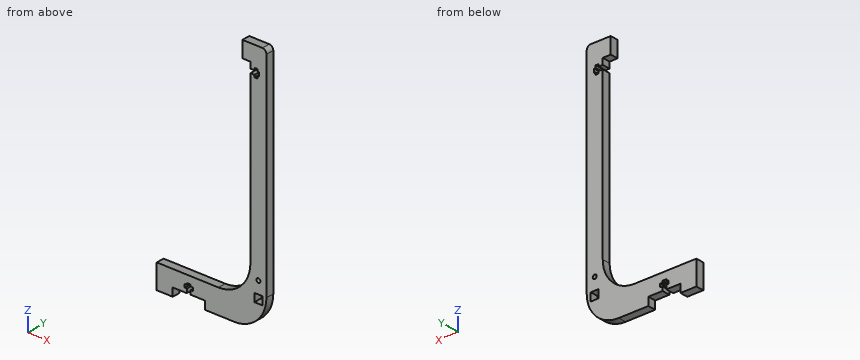
from build123d import *

# Parameters (mm, degrees)
SKETCH1_R           = 1.5875
BOSS_EXTRUDE1_DEPTH = 6.35


with BuildPart() as part:
    # Sketch1 → Boss-Extrude1 (new body)
    with BuildSketch(Plane(origin=(0, 0, 0), x_dir=(1, 0, 0), z_dir=(0, 1, 0))):
        with BuildLine():
            Line((7.882687692, 29.208698466), (-41.012312308, 29.208698466))
            Line((-41.012312308, 29.208698466), (-41.012312308, 48.258698466))
            Line((-41.012312308, 48.258698466), (-28.312312308, 48.258698466))
            Line((-28.312312308, 48.258698466), (-28.312312308, 41.908698466))
            Line((-28.312312308, 41.908698466), (-17.136241986, 41.908698466))
            Line((-17.136241986, 41.908698466), (-17.136241986, 38.733698466))
            Line((-17.136241986, 38.733698466), (-18.888841986, 38.733698466))
            Line((-18.888841986, 38.733698466), (-18.888841986, 36.193698466))
            Line((-18.888841986, 36.193698466), (-17.136241986, 36.193698466))
            Line((-17.136241986, 36.193698466), (-17.136241986, 34.923698466))
            Line((-17.136241986, 34.923698466), (-14.08838263, 34.923698466))
            Line((-14.08838263, 34.923698466), (-14.08838263, 36.193698466))
            Line((-14.08838263, 36.193698466), (-12.33578263, 36.193698466))
            Line((-12.33578263, 36.193698466), (-12.33578263, 38.733698466))
            Line((-12.33578263, 38.733698466), (-14.08838263, 38.733698466))
            Line((-14.08838263, 38.733698466), (-14.08838263, 41.908698466))
            Line((-14.08838263, 41.908698466), (-2.912312308, 41.908698466))
            Line((-2.912312308, 41.908698466), (-2.912312308, 48.258698466))
            Line((-2.912312308, 48.258698466), (20.582687692, 48.258698466))
            ThreePointArc((20.582687692, 48.258698466), (38.543199934, 40.819210709), (45.982687692, 22.858698466))
            Line((45.982687692, 22.858698466), (45.982687692, -143.587501534))
            ThreePointArc((45.982687692, -143.587501534), (45.052751722, -145.832565564), (42.807687692, -146.762501534))
            Line((42.807687692, -146.762501534), (33.282687692, -146.762501534))
            Line((33.282687692, -146.762501534), (26.932687692, -146.762501534))
            Line((26.932687692, -146.762501534), (26.932687692, -134.062501534))
            Line((26.932687692, -134.062501534), (33.282687692, -134.062501534))
            Line((33.282687692, -134.062501534), (33.282687692, -129.236431212))
            Line((33.282687692, -129.236431212), (36.457687692, -129.236431212))
            Line((36.457687692, -129.236431212), (36.457687692, -130.989031212))
            Line((36.457687692, -130.989031212), (38.997687692, -130.989031212))
            Line((38.997687692, -130.989031212), (38.997687692, -129.236431212))
            Line((38.997687692, -129.236431212), (40.267687692, -129.236431212))
            Line((40.267687692, -129.236431212), (40.267687692, -126.188571855))
            Line((40.267687692, -126.188571855), (38.997687692, -126.188571855))
            Line((38.997687692, -126.188571855), (38.997687692, -124.435971855))
            Line((38.997687692, -124.435971855), (36.457687692, -124.435971855))
            Line((36.457687692, -124.435971855), (36.457687692, -126.188571855))
            Line((36.457687692, -126.188571855), (33.282687692, -126.188571855))
            Line((33.282687692, -126.188571855), (33.282687692, -121.362501534))
            Line((33.282687692, -121.362501534), (33.282687692, 3.808698466))
            ThreePointArc((33.282687692, 3.808698466), (25.843199934, 21.769210709), (7.882687692, 29.208698466))
        make_face()
        with Locations(Location((39.632687692, 13.333698466, 0), (0, 0, 270))):
            Circle(SKETCH1_R, mode=Mode.SUBTRACT)
        Polygon((39.632687692, 29.208698466), (42.807687692, 29.208698466), (42.807687692, 22.858698466), (36.457687692, 22.858698466), (36.457687692, 29.208698466), align=None, mode=Mode.SUBTRACT)
    extrude(amount=BOSS_EXTRUDE1_DEPTH)


solid = part.part
Verification items for the finished model (mm, model axes). Coordinates: 2 decimals unless noted, no trailing zeros. Loops run counter-clockwise (first coordinate to the right, second up) from the corner with the lowest first, then second, coordinate; pieces in that order, holes last. Notation, with made-up numbers: (55.5, 85) -> (98.5, 85) arc R22 ccw to (98.5, 95) -> close; hole circle Ø9 at (-24, -22). An arc over 180 degrees is marked (long way). Answer as CSV lines item,"result".
1) Thickness scan on L1, parallel to Z at x = 40, y = 2; L2, parallel to Z at x = -14, y = 4.75; L3, parallel to Z at x = 28.5, y = 4.75. Record the ranges inside material, lowest first. Write a range as from..to.
Found:
L1,"z = -39.23..-29.21, -22.86..-14.88, -11.79..126.19, 129.24..146.76"
L2,"z = -41.91..-38.73, -36.19..-29.21"
L3,"z = -46.99..-18.64, 134.06..146.76"
2) Depth check by flat-ended pin: pin 1 (1 mm diameter, centred on y = 5, z = 62.5, fed in from -X); pin 2 (1.5 mm diameter, centred on x = -16, y = 2, fed in from -Z); pin 3 (0.9 mm diameter, centred on x = -13, y = 4, fed in from +Z); pin 4 (6 mm diameter, centred on x = -22, z = -26, fed in from +Y). Enter the tip coordinate at first touch or a pass-through.
Found:
pin 1,"stops at x = 33.28"
pin 2,"stops at z = -34.92"
pin 3,"stops at z = -29.21"
pin 4,"passes through"
3) Cross-section at C-C, the plane z = 38.5. Record the cut outline in (x, y), then the cut area to 3 significant figures.
Found:
outline,"(33.28, 0) -> (45.98, 0) -> (45.98, 6.35) -> (33.28, 6.35) -> close"
area,"80.6 mm2"
4) Cross-section at A-A, the plane z = -26. Record the cut outline in (x, y).
Found:
outline,"(20.24, 0) -> (36.46, 0) -> (36.46, 6.35) -> (20.24, 6.35) -> close; (42.81, 0) -> (45.79, 0) -> (45.79, 6.35) -> (42.81, 6.35) -> close"
5) Cross-section at B-B, the plane x = -30.5. Record the cut outline in (y, z).
Found:
outline,"(0, -48.26) -> (6.35, -48.26) -> (6.35, -29.21) -> (0, -29.21) -> close"
6) Cross-section at D-D, the plane y = 4. Count the separate pieces of the cut face and the enclosed holes in it, then the cut area to 3 significant figures.
Found:
separate pieces,"1"
enclosed holes,"2"
area,"3,700 mm2"
